Answer from the drawing. Dimensions are ordinates in mm from the lowest x, y and z of the part. Coordinates: 2 decimals unless noted, no trailing zeros. Order: outer loops, then holes, each group sorted by start corner. A loop starts at its lowest first (then second) coordinate and runs counter-clockwise, first axis right, second up. Notation, with made-up numbers: (87.5, 55.25) -> (143.5, 55.25) arc R12 ccw to (143.5, 67.25) -> close; hole circle Ø2 at (68.5, 35.25). An arc over 180 degrees is marked (long way). Answer as a JSON object with one key per item and string values. Group by question number.
1) Consider L1, parallel to Z at x = 2.5, y = 162. Determine where the line is inside the solid, lowest interval first.
2) Given pin 1 (5.5 mm diameter, centred on y = 190.5, z = 481.5, fed in from -X); pin 2 (10 mm diameter, centred on x = 2.5, y = 84.5, fed in from -Z); pin 3 (2.5 mm diameter, centred on x = 6, y = 217, fed in from +Z), each flat-ended and moving along its own axis, determine where each tip first touches the part or whether it passes through.
3) Section A-A on y = 30.5 is taken. Determine the outline of the cut face in (x, z).
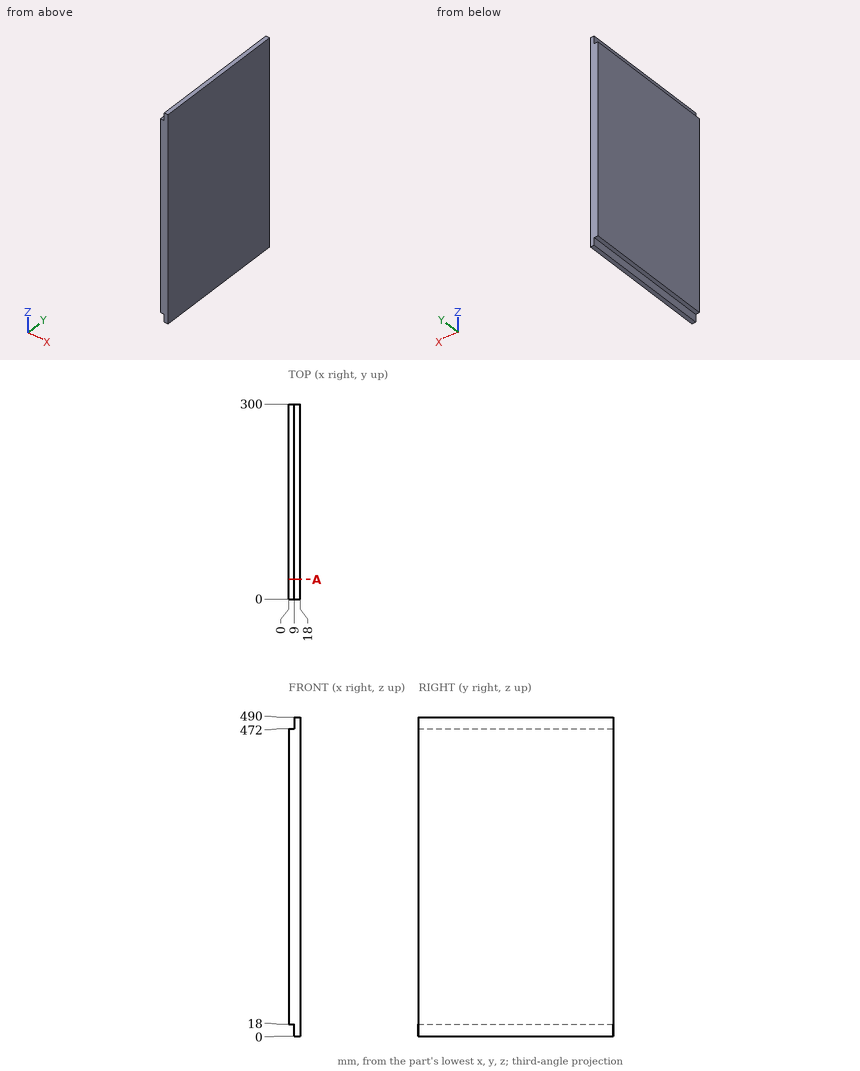
Worked answers:
{
 "1": {"L1": "z = 18 to 472"},
 "2": {"pin 1": "stops at x = 9", "pin 2": "stops at z = 18", "pin 3": "stops at z = 472"},
 "3": {"outline": "(0, 18) -> (9, 18) -> (9, 0) -> (18, 0) -> (18, 490) -> (9, 490) -> (9, 472) -> (0, 472) -> close"}
}
